Check sheet for the modelled part. Datum: model origin and axes. Units: mm. A direction names the side the tool comes from. Give positions to 0.01 mm unless a question says otherwise; leave off trailing zeros. Order: outer loops, then holes, each group sorted by start corner. A loop starts at its lowest first (then second) coordinate and runs counter-clockwise, first axis right, second up.
```python
from build123d import *

# Parameters (mm, degrees)
F0_W     = 50.8
F0_H     = 14.732
F0_R     = 3.175
F1_DEPTH = 3.175
F0_H_2   = 12.7
F2_DEPTH = 3.175
F3_SIZE2 = 1.27
F3_SIZE  = 1.27
F4_SIZE2 = 1.27
F4_SIZE  = 1.27


with BuildPart() as f1:
    # F0 (on Front) → F1 (new body, symmetric)
    with BuildSketch(Plane.XZ):
        Rectangle(F0_W, F0_H)
        with Locations((-12.7, 0)):
            Circle(F0_R, mode=Mode.SUBTRACT)
        with Locations((12.7, 0)):
            Circle(F0_R, mode=Mode.SUBTRACT)
    extrude(amount=F1_DEPTH, both=True)

    # F0 (on Front) → F2 (join)
    with BuildSketch(Plane.XZ):
        with Locations((0, -13.716)):
            Rectangle(F0_W, F0_H_2)
    extrude(amount=-F2_DEPTH)

    # F3
    f3_edges = [f1.edges().sort_by_distance(p)[0] for p in [
        (9.525, 3.175, 0),
    ]]
    chamfer(f3_edges, length=F3_SIZE, length2=F3_SIZE2)

    # F4
    f4_edges = [f1.edges().sort_by_distance(p)[0] for p in [
        (-15.875, 3.175, 0),
    ]]
    chamfer(f4_edges, length=F4_SIZE, length2=F4_SIZE2)


solid = f1.part
```
(1) Sectioned sample at A-A (x = 12.7). Enter the section's corners in (y, z) (3 decimals), plus the area to 3 significant figures.
(2) Release check for a two-part mould opening along Z. For faces 3 (the face through (0, 2, -20.066)), 4 (the face through (0, 0, 7.366)), 5 (the face through (-9.67, -0.6, 0.95)) record: released by +Z, released by -Z, zero draft, split by the parting line, or undercut.
(3) Go/stop test with flat-tipped pins: P1, Ø10, axis at x = 7.5, z = -11.5, coming from the -Y side (3 decimals); P2, Ø3.5, axis at x = -3, y = -2, coming from the -Z side. Record where each tip stops, or that it passes through.
(4) Sectioned sample at D-D (x = 6). Enter the section's corners in (y, z) (3 decimals).
(5) Sectioned sample at B-B (z = 0). Enter the section's corners in (x, y) (3 decimals).
(6) Thickness scan on L1, parallel to Z at x = -12.7, y = -2.1 (3 decimals); L2, parallel to Y at x = 9, z = -14.25 (3 decimals); L3, parallel to Z at x = -18, y = -1.75. Record the ranges inside material, lowest first.
(7) Sectioned sample at C-C (y = -2.5). Enter the section's corners in (x, z) (3 decimals).
(8) Tool access check on faces 1 (the face through (-25.4, 1, -3)), 2 (the face through (0, -2, -7.366)). Record the directions out of +Z, -Z, +X, -X, +Y, -Y that give a thin tool (end or side, any length) a straight path to the whole face; none if there is none.
Values follow:
1. outline: (-3.175, -7.366) - (0, -7.366) - (0, -20.066) - (3.175, -20.066) - (3.175, -4.445) - (1.905, -3.175) - (-3.175, -3.175) - close; (-3.175, 3.175) - (1.905, 3.175) - (3.175, 4.445) - (3.175, 7.366) - (-3.175, 7.366) - close
1. area: 91.9 mm2
2. face 3: released by -Z
2. face 4: released by +Z
2. face 5: undercut
3. P1: stops at y = -3.175
3. P2: stops at z = -7.37
4. outline: (-3.175, -7.366) - (0, -7.366) - (0, -20.066) - (3.175, -20.066) - (3.175, 7.366) - (-3.175, 7.366) - close
5. outline: (-25.4, -3.175) - (-15.875, -3.175) - (-15.875, 1.905) - (-17.145, 3.175) - (-25.4, 3.175) - close; (-9.525, -3.175) - (9.525, -3.175) - (9.525, 1.905) - (8.255, 3.175) - (-8.255, 3.175) - (-9.525, 1.905) - close; (15.875, -3.175) - (25.4, -3.175) - (25.4, 3.175) - (17.145, 3.175) - (15.875, 1.905) - close
6. L1: z = -7.366 to -3.175, 3.175 to 7.366
6. L2: y = 0 to 3.175
6. L3: z = -7.37 to 7.37
7. outline: (-25.4, -7.366) - (25.4, -7.366) - (25.4, 7.366) - (-25.4, 7.366) - close; hole circle Ø6.35 at (-12.7, 0); hole circle Ø6.35 at (12.7, 0)
8. face 1: +Z, -Z, -X, +Y, -Y
8. face 2: -Z, +X, -X, -Y
